Check sheet for the drawn part. Datum: minimum x, y, z corner. Units: mm. Round coordinates to 2 decimals unless told otherwise and drop trailing zeros. Write each loop counter-clockwise with the first axis right and the second up, starting at its lowest first coordinate (ties: lowest second). Pieces come first, ordered by that corner, then holes. Notation, with made-up numbers: (17.25, -7.5) - (75.25, -7.5) arc R13 cw to (75.25, 8.5) - close; hole circle Ø7 at (42.25, 36.5). An arc over 180 degrees is marked (long way). Return JSON: item names as keys, results as strings. Group by question number.
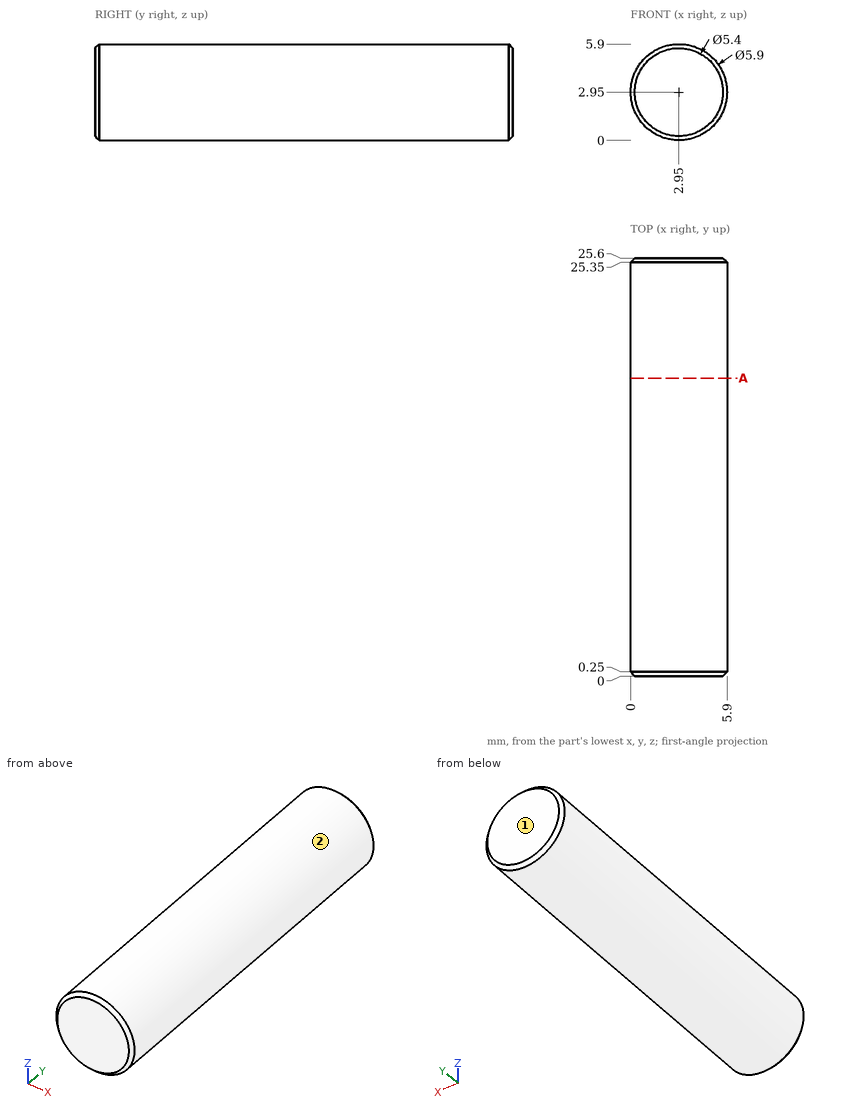
1. Mould release check, pull along Z, two halves, no side actions. Record for the marked faces 1 and 2: pulls with the +Z half, pulls with the -Z half, needs draft (parallel to the pull), parting line crosses it, or undercut.
2. Material ranges on line 1 along X through (y, z) = (24.5, 3.1); line 2 along X through (y, z) = (22.75, 1.75), recorded low to high.
3. Depth check by flat-ended pin: pin 1 Ø1 at (x, y) = (4.5, 15) entering from +Z; pin 2 Ø1 at (x, y) = (5, 6) entering from -Z. Enter the tip coordinate at first touch or a pass-through.
4. Section check A-A (y = 18.25). Enter the section's corners in (x, z).
Result sheet:
{
 "1": {"face 1": "needs draft", "face 2": "parting line crosses it"},
 "2": {"line 1": "x = 0 to 5.9", "line 2": "x = 0.26 to 5.64"},
 "3": {"pin 1": "stops at z = 5.71", "pin 2": "stops at z = 0.44"},
 "4": {"outline": "circle Ø5.9 at (2.95, 2.95)"}
}
